Autodesk Inventor part; units mm, degrees
ref_plane "YZ Plane" through (0, 0, 0) normal (1, 0, 0) x (0, 1, 0)
ref_plane "XZ Plane" through (0, 0, 0) normal (0, 1, 0) x (-1, 0, 0)
ref_plane "XY Plane" through (0, 0, 0) normal (0, 0, 1) x (1, 0, 0)
sketch "Sketch1" plane through (0, 0, 0) normal (0, 0, 1) x (1, 0, 0)
  line L0 (-10, 22.5) -> (10, 22.5)
  line L1 (10, 22.5) -> (10, -22.5)
  line L2 (10, -22.5) -> (-10, -22.5)
  line L3 (-10, -22.5) -> (-10, 22.5)
  point P0 (0, 0)
  point P1 (0, 22.5)
  point P2 (-10, 0)
  dimension "d0" = 20
  dimension "d1" = 45
extrude "Extrusion1" add sketch "Sketch1" along normal blind 30
sketch "Sketch3" plane through (0, 0, 0) normal (0, 0, -1) x (-1, 0, 0)
  circle A0 centre (-2.5, 0) radius 5
  line L0 (-10, -22.5) -> (-10, 22.5)
  point P0 (-10, 0)
  dimension "d4" = 10
  dimension "d5" = 7.5
extrude "Extrusion2" cut sketch "Sketch3" against normal through all
sketch "Sketch4" plane through (10, -22.5, 0) normal (1, 0, 0) x (0, 0, -1)
  circle A0 centre (-7, 40) radius 2.75
  circle A1 centre (-7, 5) radius 2.75
  line L0 (0, 0) -> (0, 45)
  line L1 (0, 45) -> (-30, 45)
  line L2 (0, 0) -> (-30, 0)
  circle A2 centre (-23, 40) radius 2.75
  circle A3 centre (-23, 5) radius 2.75
  line L3 (-30, 0) -> (-30, 45)
  point P0 (0, 22.5)
  dimension "d8" = 5.5
  dimension "d9" = 5.5
  dimension "d10" = 7
  dimension "d11" = 5
  dimension "d12" = 5
  dimension "d13" = 7
  dimension "d16" = 35
  dimension "d17" = 16
extrude "Extrusion3" cut sketch "Sketch4" against normal through all contours A1
pattern_linear "Rectangular Pattern1" count 2 spacing 16 along (0, 0, 1) count 2 spacing 35 along (0, 1, 0) of "Extrusion3"
sketch "Sketch5" plane through (-10, -22.5, 0) normal (0, -1, 0) x (1, 0, 0)
  line L0 (0, 0) -> (0, 30)
  line L1 (0, 0) -> (20, 0)
  point P0 (12.5, 15)
  point P1 (0, 15)
  point P2 (10, 0)
  dimension "d38" = 12.5
hole "Hole1" at (2.5, -22.5, 15) direction (0, 1, 0) diameter 4.134 end through all
equation "\"d13\" = d10"
properties part number "0005-10-015 suport tija" material "Wood (Maple)"
Read the model definition and answer for the solid it produces. Units are mm, in the model's axes. Coordinates: 2 decimals unless noted, no trailing zeros. Write each loop counter-clockwise with the first axis right and the second up, starting at its lowest first coordinate (ties: lowest second). Pieces come first, ordered by that corner, then holes. Notation, with made-up numbers: (51.25, 31.5) -> (102.25, 31.5) arc R17 ccw to (102.25, 47.5) -> close; hole circle Ø7 at (-36.75, -3). An arc over 180 degrees is marked (long way). Return JSON: item names as keys, results as strings.
(1) Consider line 1 along Y through (x, z) = (-2.75, 23); line 2 along Y through (x, z) = (5.5, 22); line 3 along Z through (x, y) = (2.5, -8.5). Determine where each line is inside the solid, lowest interval first. Write a range as from..to.
Answers below:
{"line 1": "-22.5..-20.25, -14.75..14.75, 20.25..22.5", "line 2": "-22.5..-20.06, -14.94..-4, 4..14.94, 20.06..22.5", "line 3": "0..12.93, 17.07..30"}
(2) The part is cut by section C-C on z = 7. Give the vertices of the cut face in (x, y), then the cut area to 3 significant figures.
Answers below:
{"outline": "(-10, -22.5) -> (10, -22.5) -> (10, -20.25) -> (-10, -20.25) -> close; (-10, -14.75) -> (10, -14.75) -> (10, 14.75) -> (-10, 14.75) -> close; (-10, 20.25) -> (10, 20.25) -> (10, 22.5) -> (-10, 22.5) -> close; hole circle Ø10 at (2.5, 0)", "area": "601 mm^2"}
(3) This flat-tipped pin is pushed along its axis until it touches: P1, Ø9, axis at x = 2.5, y = 0, coming from the +Z side. Where does it stop, or does it pass through?
Answers below:
{"P1": "through"}
(4) The part is cut by section B-B on x = 2.5. Give the vertices of the cut face in (y, z), then the cut area to 3 significant figures.
Answers below:
{"outline": "(-22.5, 0) -> (-5, 0) -> (-5, 12.93) -> (-22.5, 12.93) -> close; (-22.5, 17.07) -> (-5, 17.07) -> (-5, 30) -> (-22.5, 30) -> close; (5, 0) -> (22.5, 0) -> (22.5, 12.93) -> (5, 12.93) -> close; (5, 17.07) -> (22.5, 17.07) -> (22.5, 30) -> (5, 30) -> close; hole circle Ø5.5 at (-17.5, 7); hole circle Ø5.5 at (-17.5, 23); hole circle Ø5.5 at (17.5, 7); hole circle Ø5.5 at (17.5, 23)", "area": "810 mm^2"}
(5) The part is cut by section D-D on y = 3. Give the vertices of the cut face in (x, z).
Answers below:
{"outline": "(-10, 0) -> (-1.5, 0) -> (-1.5, 30) -> (-10, 30) -> close; (6.5, 0) -> (10, 0) -> (10, 30) -> (6.5, 30) -> close"}
(6) The part is cut by section A-A on y = -17.5. Give the vertices of the cut face in (x, z).
Answers below:
{"outline": "(-10, 0) -> (10, 0) -> (10, 4.25) -> (-10, 4.25) -> close; (-10, 9.75) -> (10, 9.75) -> (10, 20.25) -> (-10, 20.25) -> close; (-10, 25.75) -> (10, 25.75) -> (10, 30) -> (-10, 30) -> close; hole circle Ø4.13 at (2.5, 15)"}
(7) For a pull along X with two mould halves and no side action, classify faces 1 (the cylindrical face through (-2.27, 1.5, 14.79)), 2 (the flat face through (-5, 0, 30)), 3 (the flat face through (10, 0, 15)) as pulls with the +X half, pulls with the -X half, needs draft (parallel to the pull), parting line crosses it, or undercut.
Answers below:
{"face 1": "undercut", "face 2": "needs draft", "face 3": "pulls with the +X half"}
